Part model, mm, in its own coordinate system. Give positions to 0.01 mm unless a question says otherwise; leave off trailing zeros. Write each loop counter-clockwise with the first axis right and the second up, starting at its lowest first coordinate (ties: lowest second). Pieces come first, ordered by that corner, then holes.
from build123d import *

# Parameters (mm, degrees)
F0_W     = 927.1
F0_H     = 127
F1_DEPTH = 19.05
F2_W     = 927.1
F2_H     = 19.05
F3_DEPTH = 6.35
F4_R     = 1.5875
F5_DEPTH = 19.051


with BuildPart() as f1:
    # F0 (on Front) → F1 (new body)
    with BuildSketch(Plane.XZ):
        with Locations((463.55, -63.5)):
            Rectangle(F0_W, F0_H)
    extrude(amount=-F1_DEPTH)

    # F2 (on Front) → F3 (cut)
    with BuildSketch(Plane.XZ):
        with Locations((463.55, -111.125)):
            Rectangle(F2_W, F2_H)
    extrude(amount=-F3_DEPTH, mode=Mode.SUBTRACT)

    # F4 (on Front) → F5 (cut, through all)
    with BuildSketch(Plane.XZ):
        with Locations((19.05, -111.125)):
            Circle(F4_R)
        with Locations((196.85, -111.125)):
            Circle(F4_R)
        with Locations((374.65, -111.125)):
            Circle(F4_R)
        with Locations((552.45, -111.125)):
            Circle(F4_R)
        with Locations((730.25, -111.125)):
            Circle(F4_R)
        with Locations((908.05, -111.125)):
            Circle(F4_R)
    extrude(amount=-F5_DEPTH, mode=Mode.SUBTRACT)


solid = f1.part
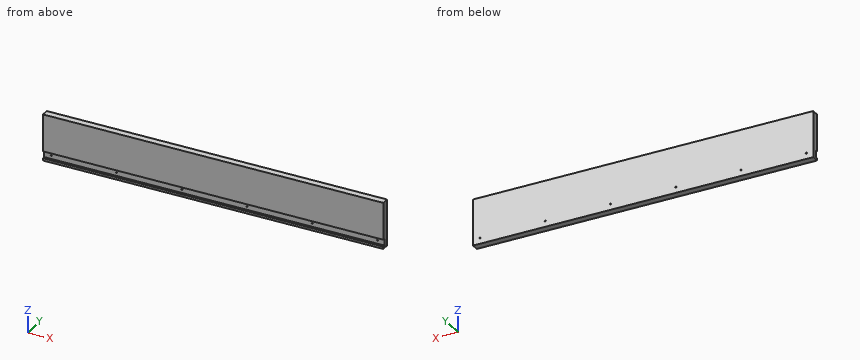
1) Flat gauge pin, fed straight in: P1, Ø4, axis at x = 19.05, z = -111.125, coming from the -Y side. Where does the tip first touch, or does it go through?
Check result:
P1: stops at y = 6.35
2) Saw through at A-A (x = 666.5). Write the cut outline in (y, z), and give its area (3 significant figures).
Check result:
outline: (0, -127) - (19.05, -127) - (19.05, 0) - (0, 0) - (0, -101.6) - (6.35, -101.6) - (6.35, -120.65) - (0, -120.65) - close
area: 2,300 mm2
3) Drill centre lines: L1, parallel to Z at x = 908.05, y = 11; L2, parallel to Z at x = 718, y = 5.5; L3, parallel to Y at x = 407, z = -116. Where is each one in solid material? Low to high.
Check result:
L1: z = -127 to -112.71, -109.54 to 0
L2: z = -127 to -120.65, -101.6 to 0
L3: y = 6.35 to 19.05
